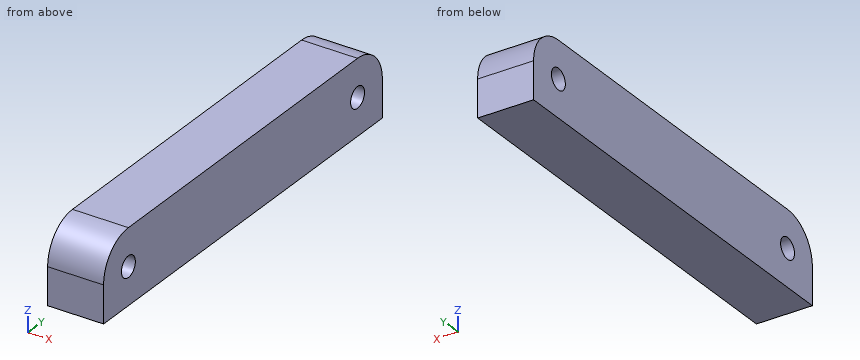
Autodesk Inventor part; units mm, degrees
ref_plane "YZ Plane" through (0, 0, 0) normal (1, 0, 0) x (0, 1, 0)
ref_plane "XZ Plane" through (0, 0, 0) normal (0, 1, 0) x (-1, 0, 0)
ref_plane "XY Plane" through (0, 0, 0) normal (0, 0, 1) x (1, 0, 0)
sketch "Sketch1" plane through (0, 0, 0) normal (1, 0, 0) x (0, 1, 0)
  circle A0 centre (0, 0) radius 1.778
  circle A1 centre (58.674, 0) radius 1.778
  line L0 (65.024, -6.35) -> (-6.35, -6.35)
  line L1 (-6.35, -6.35) -> (-6.35, 0)
  line L2 (0, 6.35) -> (58.674, 6.35)
  line L3 (65.024, 0) -> (65.024, -6.35)
  arc A2 (0, 6.35) -> (-6.35, 0) centre (0, 0) ccw
  arc A3 (65.024, 0) -> (58.674, 6.35) centre (58.674, 0) ccw
  dimension "d0" = 3.556
  dimension "d1" = 3.556
  dimension "d2" = 58.674
  dimension "d3" = 6.35
  dimension "d4" = 12.7
  dimension "d5" = 6.35
  dimension "d6" = 6.35
  dimension "d8" = 6.35
extrude "Extrusion1" add sketch "Sketch1" along normal blind 9.525
properties part number "Base"
Work out the finished part from the listing and answer in its coordinate system (mm). Round coordinates to 2 decimals unless told otherwise and drop trailing zeros. Order: outer loops, then holes, each group sorted by start corner. A loop starts at its lowest first (then second) coordinate and runs counter-clockwise, first axis right, second up.
Q1. A cutting plane is placed at B-B, the plane z = 4.75. Determine the outline of the cut face in (x, y) (3 decimals).
Solution:
outline: (0, -4.214) - (9.525, -4.214) - (9.525, 62.888) - (0, 62.888) - close
Q2. A cutting plane is placed at A-A, the plane x = 1.25. Determine the outline of the cut face in (y, z), then the cut area to 3 significant figures.
Solution:
outline: (-6.35, -6.35) - (65.02, -6.35) - (65.02, 0) arc R6.35 ccw to (58.67, 6.35) - (0, 6.35) arc R6.35 ccw to (-6.35, 0) - close; hole circle Ø3.56 at (0, 0); hole circle Ø3.56 at (58.67, 0)
area: 869 mm2
Q3. Find the intervals of material crossed by line 1 along Z through (x, y) = (5.25, 0); line 2 along Y through (x, z) = (3.5, -0.5); line 3 along Y through (x, z) = (1, -0.75), in increasing order.
Solution:
line 1: z = -6.35 to -1.78, 1.78 to 6.35
line 2: y = -6.35 to -1.71, 1.71 to 56.97, 60.38 to 65.02
line 3: y = -6.35 to -1.61, 1.61 to 57.06, 60.29 to 65.02
